CAD build for the part. Positions are in the model's coordinates, mm. Face numbers are marked on the shaded views. A direction names the side the tool comes from. Round coordinates to 2 decimals unless told otherwise and drop trailing zeros. Loops run counter-clockwise (first coordinate to the right, second up) from the corner with the lowest first, then second, coordinate; pieces in that order, holes last. Notation, with made-up numbers: M 50,83 L 71,83 A22 ccw 71,104 Z; hole C 87.25,51 d4. An arc over 180 degrees is marked long. Put each result on its own line as item: value. Start each with the question number.
Autodesk Inventor part; units mm, degrees
ref_plane "Arbeitsebene1" through (0, 0, 12) normal (0, 0, 1) x (1, 0, 0)
ref_plane "YZ Plane" through (0, 0, 0) normal (1, 0, 0) x (0, 1, 0)
ref_plane "XZ Plane" through (0, 0, 0) normal (0, 1, 0) x (-1, 0, 0)
sketch "Skizze1" plane through (0, 0, 0) normal (0, 1, 0) x (-1, 0, 0)
  line L0 (0, 0) -> (0, 12)
  line L1 (0, 12) -> (-6, 12)
  line L2 (-6, 12) -> (-6, 9)
  line L3 (-6, 9) -> (-19, 9)
  line L4 (-19, 9) -> (-19, 0)
  line L5 (-19, 0) -> (0, 0)
  dimension "d0" = 24
  dimension "d1" = 18
  dimension "d2" = 6
  dimension "d3" = 13
revolve "Umdrehung1" add sketch "Skizze1" angle 360 about axis through (19, 0, 0) along (-1, 0, 0)
sketch "Skizze2" plane through (19, 0, 0) normal (1, 0, 0) x (0, 0, -1)
  circle A0 centre (0, 0) radius 9
hole "Bohrung1" at (19, 0, 0) direction (-1, 0, 0) diameter 9 depth 19
thread "Gewinde1"
ref_plane "Arbeitsebene1" through (0, 0, 12) normal (0, 0, 1) x (1, 0, 0)
chamfer "Fasen1" distance 0.3 angle 45 2 edges at (0, 0, -12) (6, 0, -12)
properties part number "1102"
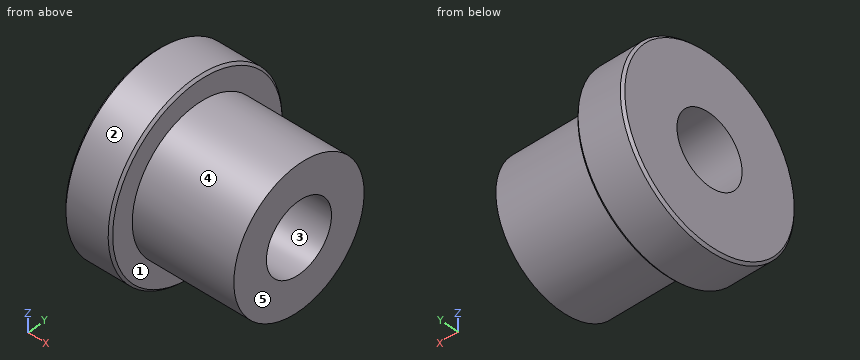
(1) Drill centre lines: line 1 along Y through (x, z) = (5, 0); line 2 along Y through (x, z) = (6.5, 0); line 3 along X through (y, z) = (7.25, -7.75). Where is each one in solid material? Low to high.
(2) Cut at D-D on x = 3.5. List the corners of the cut face in (y, z), and give its area (3 significant figures).
(3) Cut at A-A on z = 0. List the corners of the cut face in (x, y).
(4) Flat gauge pins, fed straight in: pin 1 Ø1.5 at (x, z) = (9, -6.5) entering from +Y; pin 2 Ø6 at (x, z) = (17, 8.5) entering from +Y; pin 3 Ø10 at (x, y) = (14.5, -2) entering from +Z. Where does each tip first touch, or does it go through?
(5) Mould opens along Y. For the marked faces 3, 4 and 5 say: +Y half, -Y half, draft (parallel to the pull), parting line (faces both ways), or undercut.
(6) Cut at C-C on x = 17.5. List the corners of the cut face in (y, z).
(7) Tool access for the marked faces 1 and 2: list every direction of +Z, -Z, +X, -X, +Y, -Y with a clear straight run to the whole face (end or side of a thin tool).
Taken from the geometry:
1. line 1: -12 to -4.5, 4.5 to 12
1. line 2: -9 to -4.5, 4.5 to 9
1. line 3: 0 to 6
2. outline: C 0,0 d24; hole C 0,0 d9
2. area: 389 mm2
3. outline: M 0,-11.7 L 0.3,-12 L 5.7,-12 L 6,-11.7 L 6,-9 L 19,-9 L 19,-4.5 L 0,-4.5 Z; M 0,4.5 L 19,4.5 L 19,9 L 6,9 L 6,11.7 L 5.7,12 L 0.3,12 L 0,11.7 Z
4. pin 1: y = 6.92
4. pin 2: y = 7.12
4. pin 3: z = 9
5. face 3: undercut
5. face 4: parting line
5. face 5: draft
6. outline: C 0,0 d18; hole C 0,0 d9
7. face 1: +X
7. face 2: +X, -X
